Check sheet for the drawn part. Datum: minimum x, y, z corner. Units: mm. A direction names the side the tool comes from. Round coordinates to 2 decimals unless told otherwise and drop trailing zeros. Write each loop counter-clockwise with the first axis right and the second up, starting at its lowest first coordinate (ties: lowest second). Pieces come first, ordered by that corner, then holes. Notation, with made-up numbers: (80, 71.25) - (129, 71.25) arc R28 ccw to (129, 95.25) - close; hole circle Ø8 at (34.5, 47). An arc over 180 degrees is marked (long way). Write each question's results on one line, items separated by ' | '.
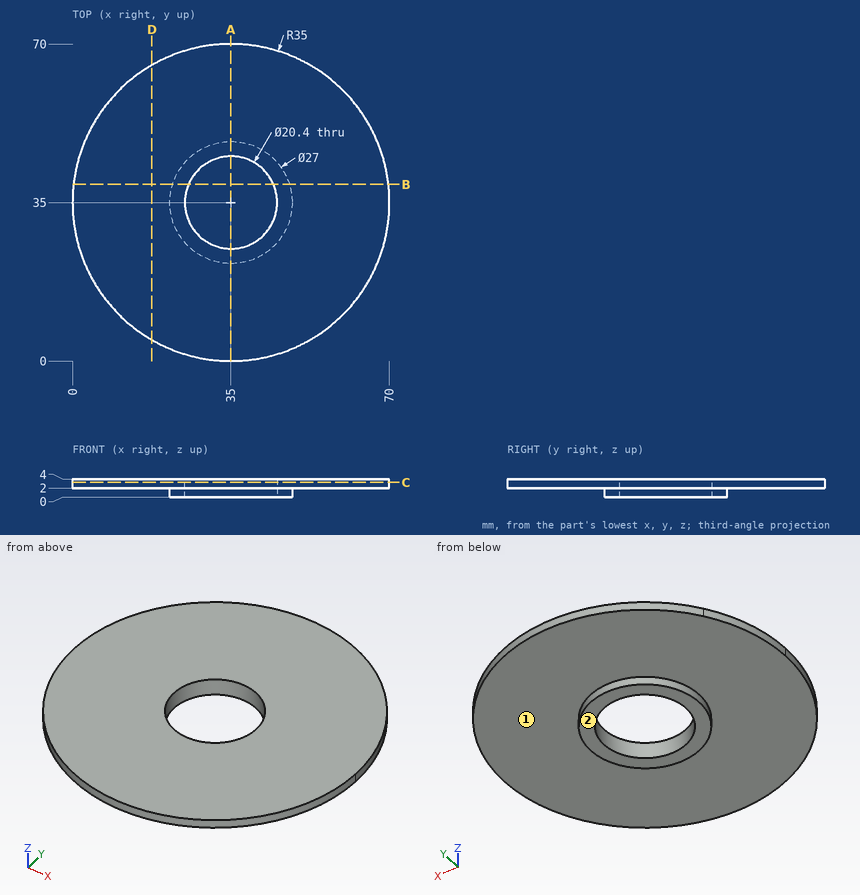
(1) Thickness scan on L1, parallel to Y at x = 35, z = 1.7; L2, parallel to Y at x = 35, z = 2.5; L3, parallel to X at y = 33.5, z = 3.8. Record the ranges inside material, lowest first.
Answer:
L1: 21.5 to 24.8, 45.2 to 48.5 | L2: 0 to 24.8, 45.2 to 70 | L3: 0.03 to 24.91, 45.09 to 69.97
(2) Go/stop test with flat-tipped pins: pin 1 Ø2 at (y, z) = (11.5, 3) entering from -X; pin 2 Ø18.5 at (x, y) = (35, 35) entering from +Z; pin 3 Ø2 at (y, z) = (46, 3) entering from -X; pin 4 Ø1.5 at (y, z) = (22.5, 1) entering from +X. Record where each tip stops, or that it passes through.
Answer:
pin 1: x = 8.19 | pin 2: through | pin 3: x = 1.46 | pin 4: x = 41.65
(3) Section check C-C (z = 3.25). Record the cut outline in (x, y).
Answer:
outline: circle Ø70 at (35, 35); hole circle Ø20.4 at (35, 35)
(4) Section check A-A (x = 35). Record the cut outline in (y, z).
Answer:
outline: (0, 2) - (21.5, 2) - (21.5, 0) - (24.8, 0) - (24.8, 4) - (0, 4) - close; (45.2, 0) - (48.5, 0) - (48.5, 2) - (70, 2) - (70, 4) - (45.2, 4) - close
(5) Section check B-B (y = 39). Record the cut outline in (x, z).
Answer:
outline: (0.23, 2) - (22.11, 2) - (22.11, 0) - (25.62, 0) - (25.62, 4) - (0.23, 4) - close; (44.38, 0) - (47.89, 0) - (47.89, 2) - (69.77, 2) - (69.77, 4) - (44.38, 4) - close
(6) Set-up check for the marked faces 1 and 2: record each of +Z, -Z, +X, -X, +Y, -Y from which the full face is reachable in a straight line by a thin tool's end or side.
Answer:
face 1: -Z | face 2: -Z, +X, -X, +Y, -Y
(7) Section check D-D (x = 17.5). Record the cut outline in (y, z), plus the area to 3 significant figures.
Answer:
outline: (4.69, 2) - (65.31, 2) - (65.31, 4) - (4.69, 4) - close | area: 121 mm2
